from build123d import *

# Parameters (mm, degrees)
BOSS_EXTRUDE1_DEPTH      = 25.4
BOSS_EXTRUDE1_DEPTH_BACK = 228.6
BOSS_EXTRUDE2_DEPTH      = 25.4


with BuildPart() as part:
    # Sketch2 → Boss-Extrude1 (new, two sides: drawn at the far end of the back side and taken through both)
    with BuildSketch(Plane.XY.offset(-BOSS_EXTRUDE1_DEPTH_BACK)):
        Polygon((-1498.565662295, -201.179604763), (-1393.765822295, -201.179604763), (-1393.800822295, -175.779604763), (-1473.165662295, -175.779604763), (-1473.165662295, -90.979604763), (-1393.790662295, -90.979604763), (-1393.740982295, -65.579604763), (-1498.565662295, -65.579604763), align=None)
    extrude(amount=BOSS_EXTRUDE1_DEPTH + BOSS_EXTRUDE1_DEPTH_BACK)

    # Sketch2<3> → Boss-Extrude2 (add)
    with BuildSketch(Plane.XY):
        Polygon((-1473.165662295, -175.779604763), (-1393.800822295, -175.779604763), (-1393.790662295, -90.979604763), (-1473.165662295, -90.979604763), align=None)
    extrude(amount=BOSS_EXTRUDE2_DEPTH)


solid = part.part
Can you work these out from the model? Positions are in its coordinate system, mm. A direction names the side the tool comes from. Give positions to 0.01 mm unless a question says otherwise; leave off trailing zeros. Loops run counter-clockwise (first coordinate to the right, second up) from the corner with the lowest first, then second, coordinate; pieces in that order, holes last. Notation, with made-up numbers: (-6.5, 72) -> (22.5, 72) arc R11 cw to (22.5, 76) -> close; hole circle Ø4 at (52, 42.5). An arc over 180 degrees is marked (long way). Write item = value, one per line.
1) Suppose I cut it at A-A on x = -1404.5. Write out the boundary of the cut face in (y, z), then the cut area to 3 significant figures.
Check result:
outline = (-201.18, -228.6) -> (-175.78, -228.6) -> (-175.78, 0) -> (-90.98, 0) -> (-90.98, -228.6) -> (-65.58, -228.6) -> (-65.58, 25.4) -> (-201.18, 25.4) -> close
area = 15,100 mm2
2) Suppose I cut it at B-B on z = -102. Write out the boundary of the cut face in (x, y), then the cut area to 3 significant figures.
Check result:
outline = (-1498.57, -201.18) -> (-1393.77, -201.18) -> (-1393.8, -175.78) -> (-1473.17, -175.78) -> (-1473.17, -90.98) -> (-1393.79, -90.98) -> (-1393.74, -65.58) -> (-1498.57, -65.58) -> close
area = 7,480 mm2
3) Thinking about a two-plate mould opening in Y: for faces 1 (the flat face through (-1498.566, -132, -103)), 2 (the flat face through (-1433, -175.78, -116)), 3 (the flat face through (-1447, -201.18, -103)), which applies, released by +Y, released by -Y, zero draft, split by the parting line, or undercut?
Check result:
face_1 = zero draft
face_2 = undercut
face_3 = released by -Y
4) Suppose I cut it at C-C on y = -138. Write out the boundary of the cut face in (x, z), then the cut area to 3 significant figures.
Check result:
outline = (-1498.57, -228.6) -> (-1473.17, -228.6) -> (-1473.17, 0) -> (-1393.8, 0) -> (-1393.8, 25.4) -> (-1498.57, 25.4) -> close
area = 8,470 mm2
5) For faces 4 (the flat face through (-1473.166, -134, -116)), 5 (the flat face through (-1445, -65.58, -103)), which set-ups out of +Z, -Z, +X, -X, +Y, -Y let a thin tool reach every point of the face, with its end or its side?
Check result:
face_4 = -Z, +X
face_5 = +Z, -Z, +X, -X, +Y
6) I need wall thicknesses on L1, parallel to Y at x = -1459, z = -4.5; L2, parallel to Z at x = -1400.5, y = -153; L3, parallel to X at y = -156.5, z = -108. Which ranges of each line are inside material? Lowest first, please. Write a range as from..to.
Check result:
L1 = -201.18..-175.78, -90.98..-65.58
L2 = 0..25.4
L3 = -1498.57..-1473.17
7) Will these pins go through, and if not, where does the flat tip stop? pin 1 (1 mm diameter, centred on y = -155.5, z = -185, fed in from +X); pin 2 (12 mm diameter, centred on y = -182, z = -41.5, fed in from +X); pin 3 (12 mm diameter, centred on x = -1447.5, y = -138.5, fed in from -Z).
Check result:
pin_1 = -1473.17
pin_2 = -1393.78
pin_3 = 0
